from build123d import *

# Parameters (mm, degrees)
SKETCH1_R                   = 70
SKETCH1_R_2                 = 30
SKETCH1_R_3                 = 3
SKETCH1_W                   = 2
SKETCH1_H                   = 5
SKETCH1_W_2                 = 22.5
SKETCH1_H_2                 = 12
SKETCH1_W_3                 = 5
SKETCH1_H_3                 = 2
Y_KSEKLIK_EKSTR_ZYON1_DEPTH = 2
SKETCH3_W                   = 2
SKETCH3_H                   = 2
SKETCH3_W_2                 = 3
BOSS_EXTRUDE1_DEPTH         = 2
SKETCH5_W                   = 5
SKETCH5_H                   = 2
CUT_EXTRUDE1_DEPTH          = 2
SKETCH6_W                   = 2
SKETCH6_H                   = 2
SKETCH6_W_2                 = 3
BOSS_EXTRUDE3_DEPTH         = 2
SKETCH8_W                   = 5
SKETCH8_H                   = 2
CUT_EXTRUDE2_DEPTH          = 2
SKETCH9_W                   = 2
SKETCH9_H                   = 2
SKETCH9_H_2                 = 3
BOSS_EXTRUDE4_DEPTH         = 2
SKETCH10_W                  = 2
SKETCH10_H                  = 2
SKETCH10_H_2                = 3
BOSS_EXTRUDE5_DEPTH         = 2
SKETCH12_W                  = 2
SKETCH12_H                  = 5
CUT_EXTRUDE4_DEPTH          = 2
SKETCH13_W                  = 2
SKETCH13_H                  = 5
CUT_EXTRUDE5_DEPTH          = 2
SKETCH14_W                  = 3
SKETCH14_H                  = 2
SKETCH14_W_2                = 2
BOSS_EXTRUDE6_DEPTH         = 2
SKETCH15_W                  = 5
SKETCH15_H                  = 2
CUT_EXTRUDE6_DEPTH          = 2
SKETCH16_W                  = 3
SKETCH16_H                  = 2
SKETCH16_W_2                = 2
BOSS_EXTRUDE9_DEPTH         = 2
SKETCH17_W                  = 5
SKETCH17_H                  = 2
CUT_EXTRUDE7_DEPTH          = 2
SKETCH18_W                  = 2
SKETCH18_H                  = 3
SKETCH18_H_2                = 2
BOSS_EXTRUDE10_DEPTH        = 2
SKETCH19_W                  = 2
SKETCH19_H                  = 5
CUT_EXTRUDE8_DEPTH          = 2


with BuildPart() as part:
    # Sketch1 → Yükseklik-Ekstrüzyon1 (new body)
    with BuildSketch(Plane(origin=(0, 0, 0), x_dir=(1, 0, 0), z_dir=(0, 1, 0))):
        with Locations(Location((0, 0, 0), (0, 0, 270))):
            Circle(SKETCH1_R)
        with Locations(Location((0, 0, 0), (0, 0, 270))):
            Circle(SKETCH1_R_2, mode=Mode.SUBTRACT)
        with Locations(Location((39.748737342, 0, 0), (0, 0, 270))):
            Circle(SKETCH1_R_3, mode=Mode.SUBTRACT)
        with Locations(Location((-39.748737342, 0, 0), (0, 0, 270))):
            Circle(SKETCH1_R_3, mode=Mode.SUBTRACT)
        with Locations(Location((0, 39.748737342, 0), (0, 0, 270))):
            Circle(SKETCH1_R_3, mode=Mode.SUBTRACT)
        with Locations((-29, 27.5)):
            Rectangle(SKETCH1_W, SKETCH1_H, mode=Mode.SUBTRACT)
        with Locations((29, 27.5)):
            Rectangle(SKETCH1_W, SKETCH1_H, mode=Mode.SUBTRACT)
        with Locations((-29, -27.5)):
            Rectangle(SKETCH1_W, SKETCH1_H, mode=Mode.SUBTRACT)
        with Locations((29, -27.5)):
            Rectangle(SKETCH1_W, SKETCH1_H, mode=Mode.SUBTRACT)
        with Locations((-39.748737342, 39.748737342)):
            Rectangle(SKETCH1_W, SKETCH1_H, mode=Mode.SUBTRACT)
        with Locations((39.748737342, 39.748737342)):
            Rectangle(SKETCH1_W, SKETCH1_H, mode=Mode.SUBTRACT)
        with Locations((39.748737342, -39.748737342)):
            Rectangle(SKETCH1_W, SKETCH1_H, mode=Mode.SUBTRACT)
        with Locations((-39.748737342, -39.748737342)):
            Rectangle(SKETCH1_W, SKETCH1_H, mode=Mode.SUBTRACT)
        with Locations((0, -39.748737342)):
            Rectangle(SKETCH1_W_2, SKETCH1_H_2, mode=Mode.SUBTRACT)
        with Locations((-64.748737342, 4)):
            Rectangle(SKETCH1_W_3, SKETCH1_H_3, mode=Mode.SUBTRACT)
        with Locations((-64.748737342, -4)):
            Rectangle(SKETCH1_W_3, SKETCH1_H_3, mode=Mode.SUBTRACT)
        with Locations((-54.748737342, -4)):
            Rectangle(SKETCH1_W_3, SKETCH1_H_3, mode=Mode.SUBTRACT)
        with Locations((-54.748737342, 4)):
            Rectangle(SKETCH1_W_3, SKETCH1_H_3, mode=Mode.SUBTRACT)
        with Locations((-4, 64.748737342)):
            Rectangle(SKETCH1_W, SKETCH1_H, mode=Mode.SUBTRACT)
        with Locations((-4, 54.748737342)):
            Rectangle(SKETCH1_W, SKETCH1_H, mode=Mode.SUBTRACT)
        with Locations((4, 54.748737342)):
            Rectangle(SKETCH1_W, SKETCH1_H, mode=Mode.SUBTRACT)
        with Locations((4, 64.748737342)):
            Rectangle(SKETCH1_W, SKETCH1_H, mode=Mode.SUBTRACT)
        with Locations((54.748737342, 4)):
            Rectangle(SKETCH1_W_3, SKETCH1_H_3, mode=Mode.SUBTRACT)
        with Locations((54.748737342, -4)):
            Rectangle(SKETCH1_W_3, SKETCH1_H_3, mode=Mode.SUBTRACT)
        with Locations((64.748737342, 4)):
            Rectangle(SKETCH1_W_3, SKETCH1_H_3, mode=Mode.SUBTRACT)
        with Locations((64.748737342, -4)):
            Rectangle(SKETCH1_W_3, SKETCH1_H_3, mode=Mode.SUBTRACT)
        with Locations((-4, -54.748737342)):
            Rectangle(SKETCH1_W, SKETCH1_H, mode=Mode.SUBTRACT)
        with Locations((4, -54.748737342)):
            Rectangle(SKETCH1_W, SKETCH1_H, mode=Mode.SUBTRACT)
        with Locations((4, -64.748737342)):
            Rectangle(SKETCH1_W, SKETCH1_H, mode=Mode.SUBTRACT)
        with Locations((-4, -64.748737342)):
            Rectangle(SKETCH1_W, SKETCH1_H, mode=Mode.SUBTRACT)
    extrude(amount=Y_KSEKLIK_EKSTR_ZYON1_DEPTH)

    # Sketch3 → Boss-Extrude1 (add)
    with BuildSketch(Plane(origin=(0, 2, 0), x_dir=(1, 0, 0), z_dir=(0, 1, 0))):
        with Locations((-66.248737342, 4)):
            Rectangle(SKETCH3_W, SKETCH3_H)
        with Locations((-53.748737342, 4)):
            Rectangle(SKETCH3_W_2, SKETCH3_H)
    extrude(amount=-BOSS_EXTRUDE1_DEPTH)

    # Sketch5 → Cut-Extrude1 (cut)
    with BuildSketch(Plane(origin=(0, 2, 0), x_dir=(1, 0, 0), z_dir=(0, 1, 0))):
        with Locations((-59.748737342, 4)):
            Rectangle(SKETCH5_W, SKETCH5_H)
    extrude(amount=-CUT_EXTRUDE1_DEPTH, mode=Mode.SUBTRACT)

    # Sketch6 → Boss-Extrude3 (add)
    with BuildSketch(Plane(origin=(0, 2, 0), x_dir=(1, 0, 0), z_dir=(0, 1, 0))):
        with Locations((-66.248737342, -4)):
            Rectangle(SKETCH6_W, SKETCH6_H)
        with Locations((-53.748737342, -4)):
            Rectangle(SKETCH6_W_2, SKETCH6_H)
    extrude(amount=-BOSS_EXTRUDE3_DEPTH)

    # Sketch8 → Cut-Extrude2 (cut)
    with BuildSketch(Plane(origin=(0, 2, 0), x_dir=(1, 0, 0), z_dir=(0, 1, 0))):
        with Locations((-59.748737342, -4)):
            Rectangle(SKETCH8_W, SKETCH8_H)
    extrude(amount=-CUT_EXTRUDE2_DEPTH, mode=Mode.SUBTRACT)

    # Sketch9 → Boss-Extrude4 (add)
    with BuildSketch(Plane(origin=(0, 2, 0), x_dir=(1, 0, 0), z_dir=(0, 1, 0))):
        with Locations((4, 66.248737342)):
            Rectangle(SKETCH9_W, SKETCH9_H)
        with Locations((4, 53.748737342)):
            Rectangle(SKETCH9_W, SKETCH9_H_2)
    extrude(amount=-BOSS_EXTRUDE4_DEPTH)

    # Sketch10 → Boss-Extrude5 (add)
    with BuildSketch(Plane(origin=(0, 2, 0), x_dir=(1, 0, 0), z_dir=(0, 1, 0))):
        with Locations((-4, 66.248737342)):
            Rectangle(SKETCH10_W, SKETCH10_H)
        with Locations((-4, 53.748737342)):
            Rectangle(SKETCH10_W, SKETCH10_H_2)
    extrude(amount=-BOSS_EXTRUDE5_DEPTH)

    # Sketch12 → Cut-Extrude4 (cut)
    with BuildSketch(Plane(origin=(0, 2, 0), x_dir=(1, 0, 0), z_dir=(0, 1, 0))):
        with Locations((-4, 59.748737342)):
            Rectangle(SKETCH12_W, SKETCH12_H)
    extrude(amount=-CUT_EXTRUDE4_DEPTH, mode=Mode.SUBTRACT)

    # Sketch13 → Cut-Extrude5 (cut)
    with BuildSketch(Plane(origin=(0, 2, 0), x_dir=(1, 0, 0), z_dir=(0, 1, 0))):
        with Locations((4, 59.748737342)):
            Rectangle(SKETCH13_W, SKETCH13_H)
    extrude(amount=-CUT_EXTRUDE5_DEPTH, mode=Mode.SUBTRACT)

    # Sketch14 → Boss-Extrude6 (add)
    with BuildSketch(Plane(origin=(0, 2, 0), x_dir=(1, 0, 0), z_dir=(0, 1, 0))):
        with Locations((53.748737342, 4)):
            Rectangle(SKETCH14_W, SKETCH14_H)
        with Locations((66.248737342, 4)):
            Rectangle(SKETCH14_W_2, SKETCH14_H)
    extrude(amount=-BOSS_EXTRUDE6_DEPTH)

    # Sketch15 → Cut-Extrude6 (cut)
    with BuildSketch(Plane(origin=(0, 2, 0), x_dir=(1, 0, 0), z_dir=(0, 1, 0))):
        with Locations((59.748737342, 4)):
            Rectangle(SKETCH15_W, SKETCH15_H)
    extrude(amount=-CUT_EXTRUDE6_DEPTH, mode=Mode.SUBTRACT)

    # Sketch16 → Boss-Extrude9 (add)
    with BuildSketch(Plane(origin=(0, 2, 0), x_dir=(1, 0, 0), z_dir=(0, 1, 0))):
        with Locations((53.748737342, -4)):
            Rectangle(SKETCH16_W, SKETCH16_H)
        with Locations((66.248737342, -4)):
            Rectangle(SKETCH16_W_2, SKETCH16_H)
    extrude(amount=-BOSS_EXTRUDE9_DEPTH)

    # Sketch17 → Cut-Extrude7 (cut)
    with BuildSketch(Plane(origin=(0, 2, 0), x_dir=(1, 0, 0), z_dir=(0, 1, 0))):
        with Locations((59.748737342, -4)):
            Rectangle(SKETCH17_W, SKETCH17_H)
    extrude(amount=-CUT_EXTRUDE7_DEPTH, mode=Mode.SUBTRACT)

    # Sketch18 → Boss-Extrude10 (add)
    with BuildSketch(Plane(origin=(0, 2, 0), x_dir=(1, 0, 0), z_dir=(0, 1, 0))):
        with Locations((-4, -53.748737342)):
            Rectangle(SKETCH18_W, SKETCH18_H)
        with Locations((-4, -66.248737342)):
            Rectangle(SKETCH18_W, SKETCH18_H_2)
        with Locations((4, -66.248737342)):
            Rectangle(SKETCH18_W, SKETCH18_H_2)
        with Locations((4, -53.748737342)):
            Rectangle(SKETCH18_W, SKETCH18_H)
    extrude(amount=-BOSS_EXTRUDE10_DEPTH)

    # Sketch19 → Cut-Extrude8 (cut)
    with BuildSketch(Plane(origin=(0, 2, 0), x_dir=(1, 0, 0), z_dir=(0, 1, 0))):
        with Locations((4, -59.748737342)):
            Rectangle(SKETCH19_W, SKETCH19_H)
        with Locations((-4, -59.748737342)):
            Rectangle(SKETCH19_W, SKETCH19_H)
    extrude(amount=-CUT_EXTRUDE8_DEPTH, mode=Mode.SUBTRACT)


solid = part.part
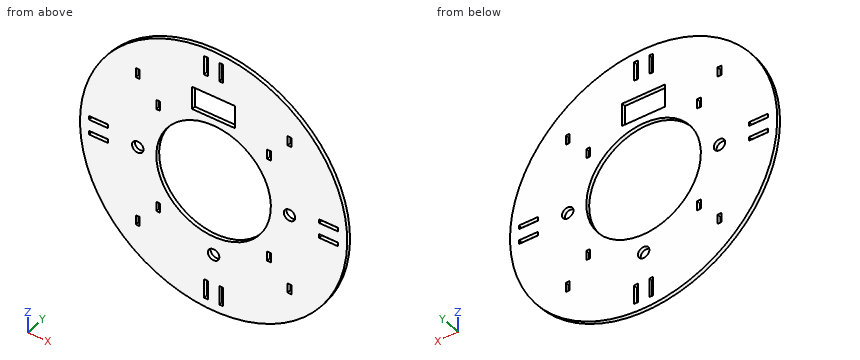
Design review of the part built by this model. Coordinates are the model's own, in mm. Give positions to 0.01 mm unless a question says otherwise; leave off trailing zeros. Order: outer loops, then holes, each group sorted by start corner. A loop starts at its lowest first (then second) coordinate and runs counter-clockwise, first axis right, second up. Notation, with made-up numbers: (87, 29.5) - (124, 29.5) arc R19 cw to (124, 47.5) - close; hole circle Ø4 at (55.5, -23.75). An arc over 180 degrees is marked (long way). Write item = value, one per line. Start each with the question number.
Q1. We need section C-C on x = -26. State the section outline as (y, z) points, plus the area to 3 significant figures.
Q2. We need section B-B on z = 0. State the section outline as (x, y) points, plus the area to 3 significant figures.
Q3. To check wall thickness, follow L1, parallel to X at y = 1.25, z = 0; L2, parallel to Z at x = -4, y = 1.45; L3, parallel to X at y = 0.95, z = 27. State the ranges of each line that lie inside material, in increasing order. Write a range as from..to.
Q4. We need section A-A on x = 0. State the section outline as (y, z) points.
Q5. We need section D-D on y = 0.4. State how many separate pieces and enclosed holes the cut face has, plus the area to 3 significant figures.
Q6. Clearance check with flat-ended pins moving along their axes: pin 1 Ø0.6 at (x, y) = (4.5, 1) entering from -Z; pin 2 Ø0.6 at (x, y) = (-60, 1) entering from +Z; pin 3 Ø1 at (x, y) = (-30, 0.5) entering from -Z. State where each tip first meets the part, or that it passes through.
Working result:
q1.outline = (0, -64.99) - (2, -64.99) - (2, -14.97) - (0, -14.97) - close; (0, 14.97) - (2, 14.97) - (2, 64.99) - (0, 64.99) - close
q1.area = 200 mm²
q2.outline = (-70, 0) - (-42.75, 0) - (-42.75, 2) - (-70, 2) - close; (-36.75, 0) - (-30, 0) - (-30, 2) - (-36.75, 2) - close; (30, 0) - (36.75, 0) - (36.75, 2) - (30, 2) - close; (42.75, 0) - (70, 0) - (70, 2) - (42.75, 2) - close
q2.area = 136 mm²
q3.L1 = -70..-42.75, -36.75..-30, 30..36.75, 42.75..70
q3.L2 = -69.89..-65.25, -55.25..-29.73, 29.73..33.75, 45.75..55.25, 65.25..69.89
q3.L3 = -64.58..-30, -28..-13.08, 13.08..28, 30..64.58
q4.outline = (0, -70) - (2, -70) - (2, -42.75) - (0, -42.75) - close; (0, -36.75) - (2, -36.75) - (2, -30) - (0, -30) - close; (0, 30) - (2, 30) - (2, 33.75) - (0, 33.75) - close; (0, 45.75) - (2, 45.75) - (2, 70) - (0, 70) - close
q5.separate_pieces = 1
q5.enclosed_holes = 21
q5.area = 12,000 mm²
q6.pin_1 = -69.87
q6.pin_2 = 36.55
q6.pin_3 = -63.48
